from build123d import *

# Parameters (mm, degrees)
EXTRUDE_1_DEPTH = 9
SKETCH_2_R      = 4
EXTRUDE_2_DEPTH = 40
CHAMFER_1_SIZE  = 0.5545


with BuildPart() as part:
    # Эскиз1 → Бобышка-Вытянуть1 (new body)
    with BuildSketch(Plane.XY):
        with BuildLine():
            ThreePointArc((6.5, 0), (-2.761654617, 5.884153616), (-4.153311931, -5))
            Line((-4.153311931, -5), (4.153311931, -5))
            ThreePointArc((4.153311931, -5), (5.884153616, -2.761654617), (6.5, 0))
        make_face()
    extrude(amount=EXTRUDE_1_DEPTH)

    # Эскиз2 → Бобышка-Вытянуть2 (add)
    with BuildSketch(Plane.XY.offset(9)):
        Circle(SKETCH_2_R)
    extrude(amount=EXTRUDE_2_DEPTH)

    # Фаска1
    chamfer_1_edges = [part.edges().sort_by_distance(p)[0] for p in [
        (-4, 0, 49),
    ]]
    chamfer(chamfer_1_edges, length=CHAMFER_1_SIZE)


solid = part.part
Here's how the part is built. I have some questions about the finished solid (model axes, mm). A direction names the side the tool comes from. Give positions to 0.01 mm unless a question says otherwise; leave off trailing zeros. Loops run counter-clockwise (first coordinate to the right, second up) from the corner with the lowest first, then second, coordinate; pieces in that order, holes last. Notation, with made-up numbers: (-25.75, 46.5) -> (-3.75, 46.5) arc R25 cw to (-3.75, 68.5) -> close; hole circle Ø10 at (-2, 23.25). An arc over 180 degrees is marked (long way). Answer as a JSON object with one key per item and string values. Group by question number.
Item 1: Imagine slicing it at C-C on y = 5.75. Write out the boundary of the cut face in (x, z), then the cut area to 3 significant figures.
Item 2: I need wall thicknesses on L1, parallel to Z at x = 4.5, y = 2.75; L2, parallel to Y at x = 0.25, z = 14.5; L3, parallel to X at y = -3.5, z = 39.5. Which ranges of each line are inside material? Lowest first, please.
Item 3: Imagine slicing it at B-B on z = 25.5. Write out the boundary of the cut face in (x, y).
Item 4: On a 3-axis mill with a long thin cutter (end or side, diameter ignored), from which of +Z, -Z, +X, -X, +Y, -Y can I reach the whole of each face in a straight line? I mean faces 1 (the flat face through (0, -5, 4)), 2 (the flat face through (3, 3, 9)). Say none if no direction works.
Item 5: Will these pins go through, and if not, where does the flat tip stop? pin 1 (4 mm diameter, centred on x = -2.5, z = 25, fed in from -Y); pin 2 (4 mm diameter, centred on y = 5.5, z = 35.5, fed in from -X); pin 3 (4 mm diameter, centred on y = -4, z = 24.5, fed in from -X).
Item 6: Imagine slicing it at A-A on x = 0. Write out the boundary of the cut face in (y, z).
Answer list:
{
 "1": {"outline": "(-3.03, 0) -> (3.03, 0) -> (3.03, 9) -> (-3.03, 9) -> close", "area": "54.6 mm2"},
 "2": {"L1": "z = 0 to 9", "L2": "y = -3.99 to 3.99", "L3": "x = -1.94 to 1.94"},
 "3": {"outline": "circle Ø8 at (0, 0)"},
 "4": {"face 1": "+Z, -Z, +X, -X, -Y", "face 2": "+Z"},
 "5": {"pin 1": "stops at y = -3.97", "pin 2": "stops at x = -1.94", "pin 3": "stops at x = -3.46"},
 "6": {"outline": "(-5, 0) -> (6.5, 0) -> (6.5, 9) -> (4, 9) -> (4, 48.45) -> (3.45, 49) -> (-3.45, 49) -> (-4, 48.45) -> (-4, 9) -> (-5, 9) -> close"}
}
